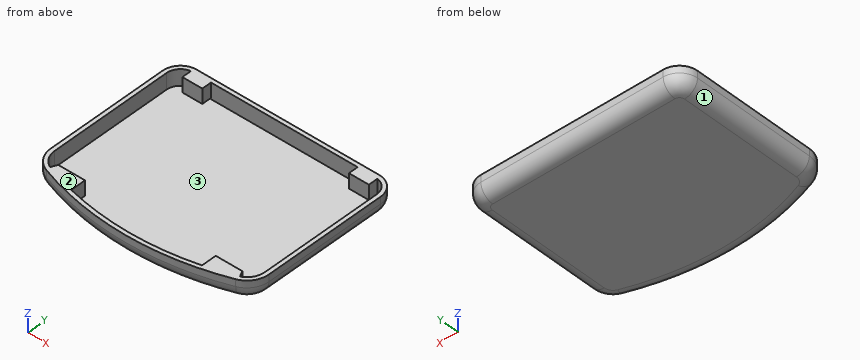
```python
from build123d import *

# Parameters (mm, degrees)
F1_DEPTH = 12.7
F2_T     = -2.54
F3_R     = 8.255
F5_W     = 12.7
F5_H     = 6.35
F6_DEPTH = 9.398


# Not quite as in the source:
# - a feature names something its author has since deleted; it is built from what else it names


with BuildPart() as f1:
    # F0 (on Top) → F1 (new body)
    with BuildSketch(Plane.XY):
        with BuildLine():
            Line((58.0965084505, 62.5356453779), (-58.0965084505, 62.5356453779))
            ThreePointArc((-58.0965084505, 62.5356453779), (-66.1787389595, 59.1878758868), (-69.5265084505, 51.1056453779))
            Line((-69.5265084505, 51.1056453779), (-69.5265084505, -27.1992570698))
            ThreePointArc((-69.5265084505, -27.1992570698), (-67.0115325937, -35.1957139026), (-60.3721316603, -40.3130159932))
            ThreePointArc((-60.3721316603, -40.3130159932), (0, -51.0474727306), (60.3721316603, -40.3130159932))
            ThreePointArc((60.3721316603, -40.3130159932), (67.0115325937, -35.1957139026), (69.5265084505, -27.1992570698))
            Line((69.5265084505, -27.1992570698), (69.5265084505, 51.1056453779))
            ThreePointArc((69.5265084505, 51.1056453779), (66.1787389595, 59.1878758868), (58.0965084505, 62.5356453779))
        make_face()
    extrude(amount=F1_DEPTH)

    # F2
    f2_openings = [f1.faces().sort_by_distance(p)[0] for p in [
        (0, 7.919531, 12.7),
    ]]
    offset(amount=F2_T, openings=f2_openings)

    # F3
    f3_edges = [f1.edges().sort_by_distance(p)[0] for p in [
        (69.526508, 11.953194, 0),
        (66.178739, 59.187876, 0),
        (0, 62.535645, 0),
        (-66.178739, 59.187876, 0),
        (-69.526508, 11.953194, 0),
        (-67.011533, -35.195714, 0),
        (0, -51.047473, 0),
        (67.011533, -35.195714, 0),
    ]]
    fillet(f3_edges, radius=F3_R)

    # F5 (on offset) → F6 (join)
    with BuildSketch(Plane.XY.offset(12.7)):
        with Locations((-53.0805146158, 57.0815077901)):
            Rectangle(F5_W, F5_H)
        with Locations((53.0805146158, 57.0815077901)):
            Rectangle(F5_W, F5_H)
        Polygon((-41.6677072644, -33.773638308), (-58.6946308613, -33.773638308), (-60.6418885291, -37.9110425711), (-53.9016760886, -40.266495198), (-41.6677072644, -43.4330925345), align=None)
        Polygon((60.6418885291, -37.9110425711), (58.6946308613, -33.773638308), (41.6677072644, -33.773638308), (41.6677072644, -43.4330925345), (53.9016760886, -40.266495198), align=None)
    extrude(amount=-F6_DEPTH)


solid = f1.part
```
For this review, take the finished solid that the model builds, in its own axes (mm). Face numbers are marked on the shaded views. Round coordinates to 2 decimals unless told otherwise and drop trailing zeros. Write each loop counter-clockwise with the first axis right and the second up, starting at its lowest first coordinate (ties: lowest second). Pieces come first, ordered by that corner, then holes. Notation, with made-up numbers: (23.5, 48) - (79.5, 48) arc R19 cw to (79.5, 71) - close; hole circle Ø9 at (-36, 56). An arc over 180 degrees is marked (long way). Answer as a JSON object with one key per item and string values.
1. Draft analysis for pull direction X (two halves, no side actions). For the marked faces 1, 2 and 3, state which applies: +X half, -X half, draft (parallel to the pull), parting line (faces both ways), or undercut.
Response values:
{"face 1": "-X half", "face 2": "draft", "face 3": "undercut"}
2. For pin 1 Ø5 at (x, z) = (41, 4) entering from -Y; pin 2 Ø6.5 at (y, z) = (57.5, 8.5) entering from -X; pin 3 Ø3 at (y, z) = (7.5, 5) entering from +X, all flat-tipped, find the tip position at first contact; note any pin that passes through.
Response values:
{"pin 1": "stops at y = -46.21", "pin 2": "stops at x = -69.09", "pin 3": "stops at x = 69.34"}
3. To check wall thickness, follow line 1 along X through (y, z) = (-22, 11.75); line 2 along X through (y, z) = (-34, 10.75); line 3 along X through (y, z) = (-36.5, 11.5). State the ranges of each line that lie inside material, in increasing order.
Response values:
{"line 1": "x = -69.53 to -66.99, 66.99 to 69.53", "line 2": "x = -67.76 to -64.74, -58.8 to -41.67, 41.67 to 58.8, 64.74 to 67.76", "line 3": "x = -65.98 to -62.2, -59.98 to -41.67, 41.67 to 59.98, 62.2 to 65.98"}
4. We need section A-A on y = 23. Give the boundary of the cut face in (x, z) (1 decimal).
Response values:
{"outline": "(-69.5, 8.3) arc R8.3 ccw to (-61.3, 0) - (61.3, 0) arc R8.3 ccw to (69.5, 8.3) - (69.5, 12.7) - (67, 12.7) - (67, 2.5) - (-67, 2.5) - (-67, 12.7) - (-69.5, 12.7) - close"}
